Input: part model. Units: mm. Frame: model coordinates. Give positions to 0.01 mm unless a question says otherwise; leave off trailing zeros. Order: outer loops, then holes, each group sorted by start corner. A loop starts at its lowest first (then second) coordinate and runs counter-clockwise, first axis right, second up. Notation, with made-up numbers: (82, 21.25) - (105, 21.25) arc R29 ccw to (105, 60.25) - close; hole circle Ø7 at (12, 64). An arc over 180 degrees is marked (long way). Answer in a Markdown table with one row per item. Add a question column.
1. Contact query for flat-ended pins moving along their axis: pin 1 (1 mm diameter, centred on x = -8, y = 1.5, fed in from +Z); pin 2 (0.6 mm diameter, centred on y = 4, z = 9, fed in from +X); pin 3 (3 mm diameter, centred on y = 3, z = 29, fed in from -X). Output: stop coordinate, or through.
2. Section query A-A on x = 0. Return loops of the section in (y, z), and give its area (3 significant figures).
3. Ray query, line 1 (Z direction, x = -8, y = 4); line 2 (X direction, y = 4.5, z = 13.5); line 3 (Z direction, x = 11, y = 5.75). Return the intervals inside material, ascending. Write a range as [from, to].
4. Section query B-B on y = 3.25. Return loops of the section in (x, z).
```python
from build123d import *

# Parameters (mm, degrees)
SKETCH1_R                 = 37.5
BOSS_EXTRUDE1_DEPTH       = 6.35
SKETCH2_R                 = 2
CUT_EXTRUDE1_DEPTH        = 2
M6X1_0_TAPPED_HOLE1_D     = 5
M6X1_0_TAPPED_HOLE1_DEPTH = 15
M6X1_0_TAPPED_HOLE1_TIP   = 1.502151548
CHAMFER1_SIZE             = 1
SKETCH6_W                 = 50.2
SKETCH6_H                 = 3.2
CUT_EXTRUDE2_DEPTH        = 10
CHAMFER2_SIZE             = 1
CUT_EXTRUDE3_DEPTH        = 18
FILLET1_R                 = 2.5


with BuildPart() as part:
    # Sketch1 → Boss-Extrude1 (new body)
    with BuildSketch(Plane(origin=(0, 0, 0), x_dir=(1, 0, 0), z_dir=(0, 1, 0))):
        with Locations(Location((0, 0, 0), (0, 0, 270))):
            Circle(SKETCH1_R)
    extrude(amount=BOSS_EXTRUDE1_DEPTH)

    # Sketch2 → Cut-Extrude1 (cut)
    with BuildSketch(Plane(origin=(0, 6.35, 0), x_dir=(1, 0, 0), z_dir=(0, 1, 0))):
        with Locations(Location((0, 30, 0), (0, 0, 270))):
            Circle(SKETCH2_R)
        with Locations(Location((5.20944533, 29.54423259, 0), (0, 0, 270))):
            Circle(SKETCH2_R)
        with Locations(Location((10.2606043, 28.190778624, 0), (0, 0, 270))):
            Circle(SKETCH2_R)
        with Locations(Location((15, 25.980762114, 0), (0, 0, 270))):
            Circle(SKETCH2_R)
        with Locations(Location((19.283628291, 22.981333294, 0), (0, 0, 270))):
            Circle(SKETCH2_R)
        with Locations(Location((22.981333294, 19.283628291, 0), (0, 0, 270))):
            Circle(SKETCH2_R)
        with Locations(Location((25.980762114, 15, 0), (0, 0, 270))):
            Circle(SKETCH2_R)
        with Locations(Location((28.190778624, 10.2606043, 0), (0, 0, 270))):
            Circle(SKETCH2_R)
        with Locations(Location((29.54423259, 5.20944533, 0), (0, 0, 270))):
            Circle(SKETCH2_R)
        with Locations(Location((30, 0, 0), (0, 0, 270))):
            Circle(SKETCH2_R)
        with Locations(Location((29.54423259, -5.20944533, 0), (0, 0, 270))):
            Circle(SKETCH2_R)
        with Locations(Location((28.190778624, -10.2606043, 0), (0, 0, 270))):
            Circle(SKETCH2_R)
        with Locations(Location((25.980762114, -15, 0), (0, 0, 270))):
            Circle(SKETCH2_R)
        with Locations(Location((22.981333294, -19.283628291, 0), (0, 0, 270))):
            Circle(SKETCH2_R)
        with Locations(Location((19.283628291, -22.981333294, 0), (0, 0, 270))):
            Circle(SKETCH2_R)
        with Locations(Location((15, -25.980762114, 0), (0, 0, 270))):
            Circle(SKETCH2_R)
        with Locations(Location((10.2606043, -28.190778624, 0), (0, 0, 270))):
            Circle(SKETCH2_R)
        with Locations(Location((5.20944533, -29.54423259, 0), (0, 0, 270))):
            Circle(SKETCH2_R)
        with Locations(Location((0, -30, 0), (0, 0, 270))):
            Circle(SKETCH2_R)
        with Locations(Location((-5.20944533, -29.54423259, 0), (0, 0, 270))):
            Circle(SKETCH2_R)
        with Locations(Location((-10.2606043, -28.190778624, 0), (0, 0, 270))):
            Circle(SKETCH2_R)
        with Locations(Location((-15, -25.980762114, 0), (0, 0, 270))):
            Circle(SKETCH2_R)
        with Locations(Location((-19.283628291, -22.981333294, 0), (0, 0, 270))):
            Circle(SKETCH2_R)
        with Locations(Location((-22.981333294, -19.283628291, 0), (0, 0, 270))):
            Circle(SKETCH2_R)
        with Locations(Location((-25.980762114, -15, 0), (0, 0, 270))):
            Circle(SKETCH2_R)
        with Locations(Location((-28.190778624, -10.2606043, 0), (0, 0, 270))):
            Circle(SKETCH2_R)
        with Locations(Location((-29.54423259, -5.20944533, 0), (0, 0, 270))):
            Circle(SKETCH2_R)
        with Locations(Location((-30, 0, 0), (0, 0, 270))):
            Circle(SKETCH2_R)
        with Locations(Location((-29.54423259, 5.20944533, 0), (0, 0, 270))):
            Circle(SKETCH2_R)
        with Locations(Location((-28.190778624, 10.2606043, 0), (0, 0, 270))):
            Circle(SKETCH2_R)
        with Locations(Location((-25.980762114, 15, 0), (0, 0, 270))):
            Circle(SKETCH2_R)
        with Locations(Location((-22.981333294, 19.283628291, 0), (0, 0, 270))):
            Circle(SKETCH2_R)
        with Locations(Location((-19.283628291, 22.981333294, 0), (0, 0, 270))):
            Circle(SKETCH2_R)
        with Locations(Location((-15, 25.980762114, 0), (0, 0, 270))):
            Circle(SKETCH2_R)
        with Locations(Location((-10.2606043, 28.190778624, 0), (0, 0, 270))):
            Circle(SKETCH2_R)
        with Locations(Location((-5.20944533, 29.54423259, 0), (0, 0, 270))):
            Circle(SKETCH2_R)
    extrude(amount=-CUT_EXTRUDE1_DEPTH, mode=Mode.SUBTRACT)

    # M6x1.0 Tapped Hole1
    with Locations(Plane(origin=(0, 6.35, 0), x_dir=(1, 0, 0), z_dir=(0, 1, 0))):
        with Locations((0, 0)):
            Hole(M6X1_0_TAPPED_HOLE1_D / 2, depth=M6X1_0_TAPPED_HOLE1_DEPTH)
            with Locations((0, 0, -(M6X1_0_TAPPED_HOLE1_DEPTH + M6X1_0_TAPPED_HOLE1_TIP / 2))):  # 118° drill point
                Cone(0, M6X1_0_TAPPED_HOLE1_D / 2, M6X1_0_TAPPED_HOLE1_TIP, mode=Mode.SUBTRACT)

    # Chamfer1
    chamfer1_edges = [part.edges().sort_by_distance(p)[0] for p in [
        (0, 6.35, -37.5),
    ]]
    chamfer(chamfer1_edges, length=CHAMFER1_SIZE)

    # Sketch6 → Cut-Extrude2 (cut)
    with BuildSketch(Plane(origin=(0, 6.35, 0), x_dir=(1, 0, 0), z_dir=(0, 1, 0))):
        with Locations((0, -9.5)):
            Rectangle(SKETCH6_W, SKETCH6_H)
    extrude(amount=-CUT_EXTRUDE2_DEPTH, mode=Mode.SUBTRACT)

    # Chamfer2
    chamfer2_edges = [part.edges().sort_by_distance(p)[0] for p in [
        (25.1, 3.175, 7.9),
        (25.1, 3.175, 11.1),
        (-25.1, 3.175, 11.1),
        (-25.1, 3.175, 7.9),
    ]]
    chamfer(chamfer2_edges, length=CHAMFER2_SIZE)

    # Sketch7 → Cut-Extrude3 (cut)
    with BuildSketch(Plane(origin=(0, 6.35, 0), x_dir=(1, 0, 0), z_dir=(0, 1, 0))):
        Polygon((-45.405269777, -5.20944533), (48.202750853, -5.20944533), (48.202750853, 45.076127107), (-45.405269777, 43.569791143), align=None)
    extrude(amount=-CUT_EXTRUDE3_DEPTH, mode=Mode.SUBTRACT)

    # Fillet1
    fillet1_edges = [part.edges().sort_by_distance(p)[0] for p in [
        (37.136392923, 2.675, 5.20944533),
        (-37.136392923, 2.675, 5.20944533),
    ]]
    fillet(fillet1_edges, radius=FILLET1_R)


solid = part.part
```
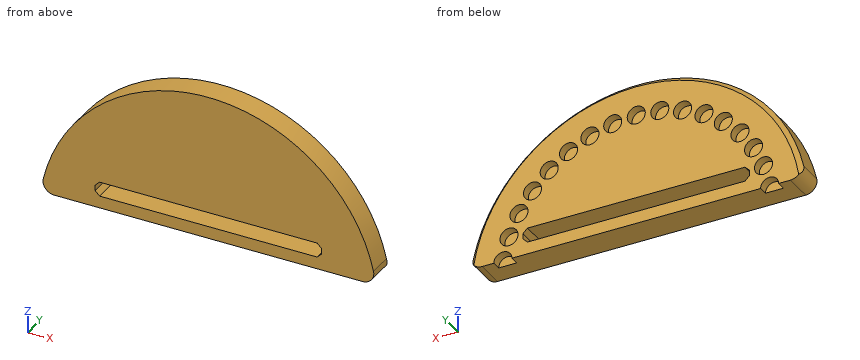
Answer:
| question | item | result |
|---|---|---|
| 1 | pin 1 | stops at z = 36.74 |
| 1 | pin 2 | stops at x = 36.48 |
| 1 | pin 3 | stops at x = -25.5 |
| 2 | outline | (0, 5.21) - (6.35, 5.21) - (6.35, 7.9) - (0, 7.9) - close; (0, 11.1) - (6.35, 11.1) - (6.35, 28) - (4.35, 28) - (4.35, 32) - (6.35, 32) - (6.35, 36.5) - (5.35, 37.5) - (0, 37.5) - close |
| 2 | area | 176 mm² |
| 3 | line 1 | z = [5.21, 7.9], [11.1, 36.64] |
| 3 | line 2 | x = [-34.99, -27.3], [-24.66, 24.66], [27.3, 34.99] |
| 3 | line 3 | z = [5.21, 7.9], [11.1, 26.33], [30.05, 35.43] |
| 4 | outline | (-36.58, 8.26) arc R2.5 ccw to (-34.14, 5.21) - (34.14, 5.21) arc R2.5 ccw to (36.58, 8.26) arc R37.5 ccw to start; hole (-25.1, 8.9) - (-24.1, 7.9) - (24.1, 7.9) - (25.1, 8.9) - (25.1, 10.1) - (24.1, 11.1) - (-24.1, 11.1) - (-25.1, 10.1) - close |
